Verification items for the finished model (mm, model axes). Coordinates: 2 decimals unless noted, no trailing zeros. Order: outer loops, then holes, each group sorted by start corner. A loop starts at its lowest first (then second) coordinate and runs counter-clockwise, first axis right, second up. Notation, with made-up numbers: M 48,20 L 100,20 A22 cw 100,27 Z; hole C 57.25,-14.5 d6. An arc over 180 degrees is marked long. Return JSON: item names as keys, results as strings.
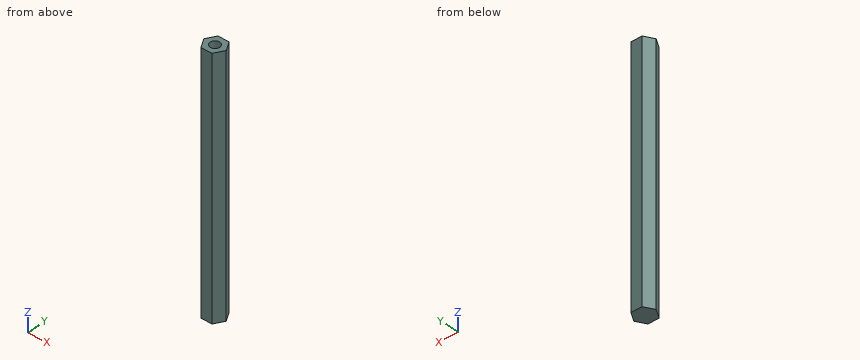
```python
from build123d import *

# Parameters (mm, degrees)
SKETCH_1_R             = 1.5
EXTRUDE_1_DEPTH        = 65
HOLE_WIZARD_M3_1_D     = 2.5
HOLE_WIZARD_M3_1_DEPTH = 7.5
HOLE_WIZARD_M3_1_TIP   = 0.751075774


with BuildPart() as part:
    # 草图1 → 凸台-拉伸1 (new body)
    # profile 1 of 2: a face of its own
    with BuildSketch(Plane.XY):
        Polygon((-1.443375673, -2.5), (1.443375673, -2.5), (2.886751346, 0), (1.443375673, 2.5), (-1.443375673, 2.5), (-2.886751346, 0), align=None)
        Circle(SKETCH_1_R, mode=Mode.SUBTRACT)
    # profile 2 of 2: a face of its own
    with BuildSketch(Plane.XY):
        Circle(SKETCH_1_R)
    extrude(amount=EXTRUDE_1_DEPTH)

    # M3 螺纹孔1
    with Locations(Plane.XY.offset(65)):
        with Locations((0, 0)):
            Hole(HOLE_WIZARD_M3_1_D / 2, depth=HOLE_WIZARD_M3_1_DEPTH)
            with Locations((0, 0, -(HOLE_WIZARD_M3_1_DEPTH + HOLE_WIZARD_M3_1_TIP / 2))):  # 118° drill point
                Cone(0, HOLE_WIZARD_M3_1_D / 2, HOLE_WIZARD_M3_1_TIP, mode=Mode.SUBTRACT)


solid = part.part
```
Q1. Go/stop test with flat-tipped pins: pin 1 (1.5 mm diameter, centred on y = -1.5, z = 56, fed in from +X); pin 2 (2 mm diameter, centred on x = 0, y = 0, fed in from +Z). Record where each tip stops, or that it passes through.
Values:
{"pin 1": "x = 2.45", "pin 2": "z = 57.35"}
Q2. Cross-section at A-A, the plane z = 59. Record the boundary of the cut face in (x, y), and give its area (3 significant figures).
Values:
{"outline": "M -2.89,0 L -1.44,-2.5 L 1.44,-2.5 L 2.89,0 L 1.44,2.5 L -1.44,2.5 Z; hole C 0,0 d2.5", "area": "16.7 mm^2"}
Q3. Cross-section at B-B, the plane z = 20.5. Record the boundary of the cut face in (x, y).
Values:
{"outline": "M -2.89,0 L -1.44,-2.5 L 1.44,-2.5 L 2.89,0 L 1.44,2.5 L -1.44,2.5 Z"}
Q4. Cross-section at C-C, the plane x = 2.1. Record the boundary of the cut face in (y, z), and give its area (3 significant figures).
Values:
{"outline": "M -1.36,0 L 1.36,0 L 1.36,65 L -1.36,65 Z", "area": "177 mm^2"}
Q5. Material ranges on line 1 along Y through (x, z) = (0, 62.75); line 2 along X through (y, z) = (0, 59.75); line 3 along X through (y, z) = (-0.9, 61), recorded low to high.
Values:
{"line 1": "-2.5 to -1.25, 1.25 to 2.5", "line 2": "-2.89 to -1.25, 1.25 to 2.89", "line 3": "-2.37 to -0.87, 0.87 to 2.37"}
